The model under review builds one solid part; all positions refer to its coordinate system, in mm. A direction names the side the tool comes from. Round coordinates to 2 decimals unless told otherwise and drop trailing zeros. Loops run counter-clockwise (first coordinate to the right, second up) from the corner with the lowest first, then second, coordinate; pieces in that order, holes last. Notation, with made-up numbers: (58, -4) -> (91, -4) arc R26 cw to (91, 27) -> close; hole circle Ø10 at (62.25, 26.25). An arc over 180 degrees is marked (long way). Write each question's results on one line, items separated by ' | '. Start each with the question number.
Item 1: Clearance check with flat-ended pins moving along their axes: pin 1 Ø1.7 at (x, z) = (12.5, 4.5) entering from -Y; pin 2 Ø4.5 at (y, z) = (-2.5, 3.5) entering from +X; pin 3 Ø6 at (x, y) = (-5.5, -9) entering from -Z; pin 4 Ø5 at (x, z) = (-5, 2.5) entering from -Y. State where each tip first meets the part, or that it passes through.
Item 2: We need section C-C (x = 0). Give the boundary of the cut face in (y, z), and give its area (3 significant figures).
Item 3: Mouldability with a two-part tool opening along Y and no side actions: class faces 1 (the flat face through (-18.95, -11, 4)), 2 (the cylindrical face through (-0.54, -2.44, 4.44)), 3 (the flat face through (-9.047, -7.902, 4.437)), 4 (the flat face through (-2.05, -12.77, 4.44)) as pulls with the +Y half, pulls with the -Y half, needs draft (parallel to the pull), parting line crosses it, or undercut.
Item 4: Tool access review of faces 5 (the flat face through (6, -5, 4)), 6 (the flat face through (7, 16.242, 4)), 7 (the flat face through (-14.474, -14.787, 4.437)), 8 (the flat face through (-15.074, -8.802, 4.437)), 9 (the flat face through (-6, -3, 4)): name each direction out of +Z, -Z, +X, -X, +Y, -Y from which nothing blocks a thin tool from reaching the whole face with its end or side.
Item 5: For L1, parallel to Y at x = 0, z = 6.75; L2, parallel to X at y = -5.5, z = 7.75; L3, parallel to Y at x = -1, z = 7.75, list the stretches that pass through material, from the lowest coordinate up. Write a range as from..to.
Item 6: We need section A-A (y = -2). Give the boundary of the cut face in (x, z), and give its area (3 significant figures).
Item 7: We need section B-B (z = 7). Give the boundary of the cut face in (x, y), and give its area (3 significant figures).
Item 8: We need section D-D (x = 12.5). Give the boundary of the cut face in (y, z), and give its area (3 significant figures).
from build123d import *

# Parameters (mm, degrees)
SKETCH_1_R      = 2.5
EXTRUDE_1_DEPTH = 9


with BuildPart() as part:
    # 스케치1 → 보스-돌출1 (new body)
    with BuildSketch(Plane.XY):
        with BuildLine():
            Line((-6, 0), (-6, -5.928252217))
            Line((-6, -5.928252217), (-12.181462163, -9.930872029))
            Line((-12.181462163, -9.930872029), (-15.181462163, -9.930872029))
            Line((-15.181462163, -9.930872029), (-14.962549322, -7.64046453))
            ThreePointArc((-14.962549322, -7.64046453), (-15.12996585, -7.275687064), (-15.529724639, -7.239856856))
            Line((-15.529724639, -7.239856856), (-18.949704861, -8.833960932))
            Line((-18.949704861, -8.833960932), (-18.949704861, -12.404351558))
            Line((-18.949704861, -12.404351558), (-18.949704861, -14.067418225))
            Line((-18.949704861, -14.067418225), (-9.871536241, -15.526817987))
            Line((-9.871536241, -15.526817987), (6, -9.930872029))
            Line((6, -9.930872029), (6, 0.655573526))
            Line((6, 0.655573526), (10.754294738, 11.24201908))
            Line((10.754294738, 11.24201908), (14.08643491, 11.24201908))
            Line((14.08643491, 11.24201908), (14.08643491, 16.24201908))
            Line((14.08643491, 16.24201908), (0.716889728, 16.24201908))
            Line((0.716889728, 16.24201908), (-5.473385983, 2.458057338))
            ThreePointArc((-5.473385983, 2.458057338), (-5.866869519, 1.256917678), (-6, 0))
        make_face()
        Circle(SKETCH_1_R, mode=Mode.SUBTRACT)
    extrude(amount=EXTRUDE_1_DEPTH)


solid = part.part
Here are the results:
1) pin 1: stops at y = 11.24 | pin 2: stops at x = 6 | pin 3: stops at z = 0 | pin 4: stops at y = -14.69
2) outline: (-12.05, 0) -> (-2.5, 0) -> (-2.5, 9) -> (-12.05, 9) -> close; (2.5, 0) -> (14.65, 0) -> (14.65, 9) -> (2.5, 9) -> close | area: 195 mm2
3) face 1: needs draft | face 2: undercut | face 3: pulls with the +Y half | face 4: pulls with the -Y half
4) face 5: +Z, -Z, +X, -Y | face 6: +Z, -Z, +X, -X, +Y | face 7: +Z, -Z, -X, -Y | face 8: +Z, -Z | face 9: +Z, -Z, -X, +Y
5) L1: y = -12.05..-2.5, 2.5..14.65 | L2: x = -6..6 | L3: y = -12.4..-2.29, 2.29..12.42
6) outline: (-6, 0) -> (-1.5, 0) -> (-1.5, 9) -> (-6, 9) -> close; (1.5, 0) -> (6, 0) -> (6, 9) -> (1.5, 9) -> close | area: 81.0 mm2
7) outline: (-18.95, -14.07) -> (-9.87, -15.53) -> (6, -9.93) -> (6, 0.66) -> (10.75, 11.24) -> (14.09, 11.24) -> (14.09, 16.24) -> (0.72, 16.24) -> (-5.47, 2.46) arc R6 ccw to (-6, 0) -> (-6, -5.93) -> (-12.18, -9.93) -> (-15.18, -9.93) -> (-14.96, -7.64) arc R0.4 ccw to (-15.53, -7.24) -> (-18.95, -8.83) -> close; hole circle Ø5 at (0, 0) | area: 418 mm2
8) outline: (11.24, 0) -> (16.24, 0) -> (16.24, 9) -> (11.24, 9) -> close | area: 45.0 mm2
